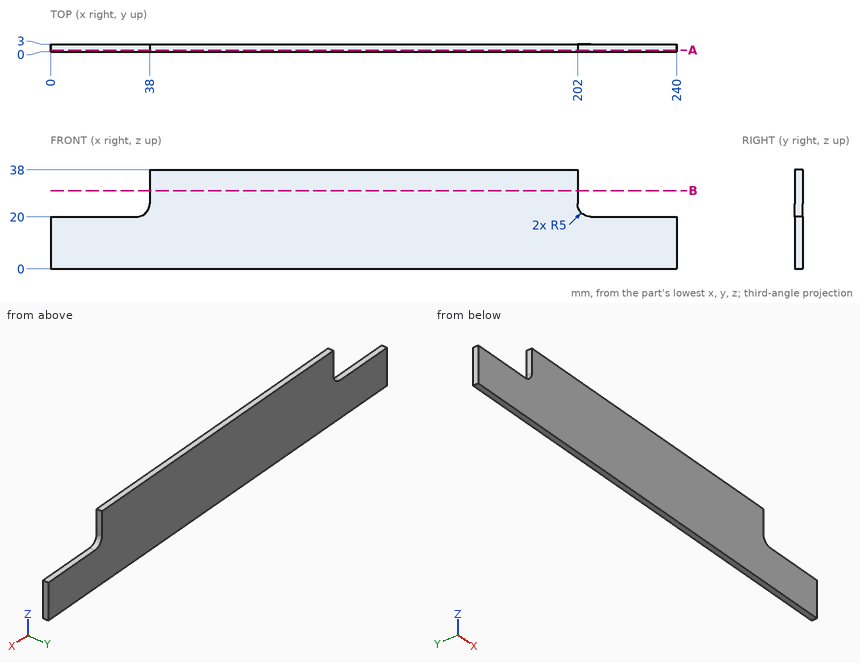
Answer from the drawing. Dimensions are ordinates in mm from the lowest x, y and z of the part. Round coordinates to 2 decimals unless told otherwise and drop trailing zeros. Loops run counter-clockwise (first coordinate to the right, second up) from the corner with the lowest first, then second, coordinate; pieces in that order, holes last. Notation, with made-up numbers: M 2.25,-34.75 L 16.25,-34.75 A22 cw 16.25,-5.75 Z; hole C 37,77.5 d3. An arc over 180 degrees is marked long. One line per question, with ' | ' between items. Start each with the question number.
(1) A cutting plane is placed at B-B on z = 30. Write down the section's boundary in (x, y).
(2) A cutting plane is placed at A-A on y = 0.65. Write down the section's boundary in (x, z).
(3) Find the intervals of material crossed by line 1 (Z direction, x = 27.5, y = 1.7); line 2 (X direction, y = 1.9, z = 36.5); line 3 (X direction, y = 0.35, z = 24), in increasing order.
(4) Flat-ended cylindrical pins translate along their axes: pin 1 Ø1 at (y, z) = (2.5, 31.5) entering from +X; pin 2 Ø1 at (y, z) = (1.5, 29.5) entering from -X. Find the tip coordinate at first contact, or state that the pin passes through.
Geometry check:
1) outline: M 38,0 L 202,0 L 202,3 L 38,3 Z
2) outline: M 0,0 L 240,0 L 240,20 L 207,20 A5 cw 202,25 L 202,38 L 38,38 L 38,25 A5 cw 33,20 L 0,20 Z
3) line 1: z = 0 to 20 | line 2: x = 38 to 202 | line 3: x = 37.9 to 202.1
4) pin 1: stops at x = 202 | pin 2: stops at x = 38
